from build123d import *

# Parameters (mm, degrees)
SKETCH1_R           = 36
BOSS_EXTRUDE1_DEPTH = 15
SKETCH2_R           = 27
BOSS_EXTRUDE2_DEPTH = 46
SKETCH3_R           = 36
BOSS_EXTRUDE3_DEPTH = 38


with BuildPart() as part:
    # Sketch1 → Boss-Extrude1 (new body)
    with BuildSketch(Plane.XY):
        with BuildLine():
            Line((-64.569893475, 47.23059238), (-34.517510455, -54.224552409))
            ThreePointArc((-34.517510455, -54.224552409), (-5.165734392, -8.372550074), (36, -44))
            ThreePointArc((36, -44), (35.627449926, -49.165734392), (34.517510455, -54.224552409))
            Line((34.517510455, -54.224552409), (64.569893475, 47.23059238))
            ThreePointArc((64.569893475, 47.23059238), (0, 80), (-64.569893475, 47.23059238))
        make_face()
        with Locations((0, -44)):
            Circle(SKETCH1_R)
    extrude(amount=BOSS_EXTRUDE1_DEPTH)

    # Sketch2 → Boss-Extrude2 (add)
    with BuildSketch(Plane.XY.offset(15)):
        with Locations((0, -44)):
            Circle(SKETCH2_R)
    extrude(amount=BOSS_EXTRUDE2_DEPTH)

    # Sketch3 → Boss-Extrude3 (add)
    with BuildSketch(Plane(origin=(0, 0, 0), x_dir=(-1, 0, 0), z_dir=(0, 0, -1))):
        Circle(SKETCH3_R)
    extrude(amount=BOSS_EXTRUDE3_DEPTH)

    # Mirror1: part across plane


with BuildPart() as part_1:
    add(part.part)
    add(part.part.mirror(Plane.XY.offset(38)))


solid = part_1.part
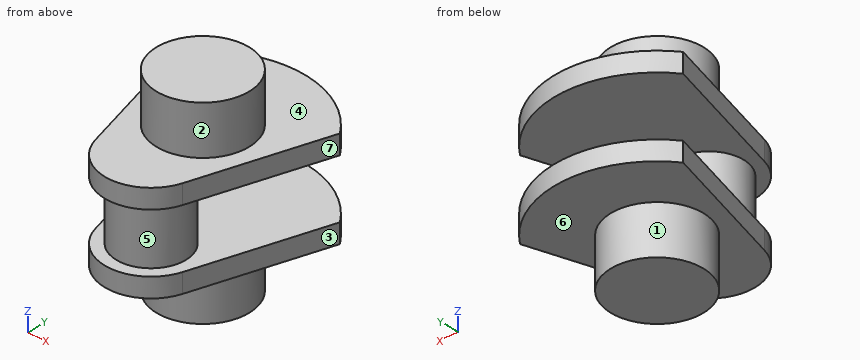
Geometry: final body of the model. Coordinates: model frame, mm. Face numbers are marked on the shaded views. A direction names the side the tool comes from. Round coordinates to 2 decimals unless told otherwise and drop trailing zeros. Loops run counter-clockwise (first coordinate to the right, second up) from the corner with the lowest first, then second, coordinate; pieces in that order, holes last.
Q1. Pull-direction query (Z, two-part tool) for the marked faces 4, 5, 6 and 7; classes: released by +Z, released by -Z, zero draft, split by the parting line, or undercut.
Q2. Section A-A on x = -54. Return loops of the section in (y, z), plus the area to 3 significant figures.
Q3. Pin query (flat end, axial travel): P1, Ø1.5, axis at x = 19.5, z = 48, coming from the -Y side; P2, Ø1, axis at y = -44, z = 57.5, coming from the +X side; P3, Ø2, axis at x = 15.5, y = -38, coming from the -Z side. Return the tip coordinate at first contact, or that it passes through.
Q4. Section C-C on x = 0. Return loops of the section in (y, z).
Q5. Material intervals for L1, parallel to Z at x = -5, y = -5.5; L2, parallel to Z at x = 28, y = -54; L3, parallel to Y at x = 0, z = 84, sorted ascending.
Q6. Section B-B on y = 0. Return loops of the section in (x, z).
Q7. Access query for the marked faces 1, 2 and 3. Directions: +Z, -Z, +X, -X, +Y, -Y. A direction counts if a zero-diameter tool reaches every point of the face in a straight line with its end or side. Return the directions, or none.
Q8. Section D-D on z = 28. Return loops of the section in (x, y).
Evaluation:
1. face 4: released by +Z
1. face 5: undercut
1. face 6: released by -Z
1. face 7: zero draft
2. outline: (11.55, 0) - (59.03, 0) - (59.03, 15) - (11.55, 15) - close; (11.55, 61) - (59.03, 61) - (59.03, 76) - (11.55, 76) - close
2. area: 1,420 mm2
3. P1: stops at y = -63.43
3. P2: stops at x = 27
3. P3: stops at z = 0
4. outline: (-80, 0) - (-36, 0) - (-36, -38) - (36, -38) - (36, 0) - (80, 0) - (80, 15) - (-17, 15) - (-17, 61) - (80, 61) - (80, 76) - (36, 76) - (36, 114) - (-36, 114) - (-36, 76) - (-80, 76) - (-80, 61) - (-71, 61) - (-71, 15) - (-80, 15) - close
5. L1: z = -38 to 15, 61 to 114
5. L2: z = 0 to 15, 61 to 76
5. L3: y = -36 to 36
6. outline: (-50.58, 0) - (-36, 0) - (-36, -38) - (36, -38) - (36, 0) - (50.58, 0) - (50.58, 15) - (-50.58, 15) - close; (-50.58, 61) - (50.58, 61) - (50.58, 76) - (36, 76) - (36, 114) - (-36, 114) - (-36, 76) - (-50.58, 76) - close
7. face 1: -Z
7. face 2: +Z
7. face 3: +Z, -Z, +X, -Y
8. outline: circle Ø54 at (0, -44)
